```python
from build123d import *
from OCP.BRepFilletAPI import BRepFilletAPI_MakeFillet

# Parameters (mm, degrees)
ESQUISSE1_W             = 23
ESQUISSE1_H             = 20
BOSS_EXTRU_1_DEPTH      = 11.5
ESQUISSE2_W             = 11.5
ESQUISSE2_H             = 1.8
BOSS_EXTRU_2_DEPTH      = 4.5
BOSS_EXTRU_3_DEPTH      = 4
ENL_V_MAT_EXTRU_1_REACH = 27.382
ESQUISSE4_R             = 0.5
CONG_1_R1               = 1
CONG_1_R2               = 2
ESQUISSE5_R             = 2
BOSS_EXTRU_4_DEPTH      = 3.5


with BuildPart() as part:
    # Esquisse1 → Boss.-Extru.1 (new body)
    with BuildSketch(Plane.XY):
        Rectangle(ESQUISSE1_W, ESQUISSE1_H)
    extrude(amount=BOSS_EXTRU_1_DEPTH)

    # Esquisse2 → Boss.-Extru.2 (add)
    with BuildSketch(Plane(origin=(11.5, 0, 0), x_dir=(0, 0, -1), z_dir=(1, 0, 0))):
        with Locations((-5.75, 5.1)):
            Rectangle(ESQUISSE2_W, ESQUISSE2_H)
    boss_extru_2 = extrude(amount=BOSS_EXTRU_2_DEPTH)

    # Sym_trie1: Boss.-Extru.2 across plane
    add(boss_extru_2.mirror(Plane(origin=(0, 0, 0), x_dir=(0, 0, 1), z_dir=(1, 0, 0))))

    # Esquisse3 → Boss.-Extru.3 (add)
    with BuildSketch(Plane(origin=(0, 10, 0), x_dir=(1, 0, 0), z_dir=(0, 1, 0))):
        with BuildLine():
            Line((-0.290992678, -8.604781917), (-0.577609195, -8.604781917))
            ThreePointArc((-0.577609195, -8.604781917), (-3.459311015, -5.723080096), (-0.577609195, -2.841378276))
            Line((-0.577609195, -2.841378276), (-0.247327135, -2.841378276))
            ThreePointArc((-0.247327135, -2.841378276), (0.608978248, -2.648791092), (1.30037019, -2.108119366))
            ThreePointArc((1.30037019, -2.108119366), (11.499942495, -5.775715864), (1.267973174, -9.351934971))
            ThreePointArc((1.267973174, -9.351934971), (0.573387477, -8.801216851), (-0.290992678, -8.604781917))
        make_face()
    extrude(amount=BOSS_EXTRU_3_DEPTH)

    # Esquisse4 → Enl_v. mat.-Extru.1 (cut, up to next)
    with BuildSketch(Plane(origin=(0, 6, 0), x_dir=(1, 0, 0), z_dir=(0, 1, 0)), mode=Mode.PRIVATE) as enl_v_mat_extru_1_sk1:
        with Locations(Location((-13.75, -5.75, 0), (0, 0, 270))):
            Circle(ESQUISSE4_R)
    enl_v_mat_extru_1_tool1 = extrude(enl_v_mat_extru_1_sk1.sketch, amount=-ENL_V_MAT_EXTRU_1_REACH, mode=Mode.PRIVATE) & part.part
    enl_v_mat_extru_1 = enl_v_mat_extru_1_tool1.solids().sort_by_distance((-13.75, 6, 5.75))[0]
    add(enl_v_mat_extru_1, mode=Mode.SUBTRACT)

    # Sym_trie2: Enl_v. mat.-Extru.1 across plane
    add(enl_v_mat_extru_1.mirror(Plane(origin=(0, 0, 0), x_dir=(0, 0, 1), z_dir=(1, 0, 0))), mode=Mode.SUBTRACT)

    # Cong_1: one fillet with a radius per group of edges: ONE call of the kernel's fillet builder (fillet() takes one radius for all edges)
    cong_1_edges_1 = [part.edges().sort_by_distance(p)[0] for p in [
        (-11.5, 8, 11.5),
        (11.5, 8, 0),
        (11.5, 8, 11.5),
        (-11.5, -2.9, 0),
        (-11.5, -2.9, 11.5),
        (11.5, -2.9, 11.5),
        (-11.5, 8, 0),
        (11.5, -2.9, 0),
    ]]
    cong_1_edges_2 = [part.edges().sort_by_distance(p)[0] for p in [
        (16, 5.1, 11.5),
        (16, 5.1, 0),
        (-16, 5.1, 0),
        (-16, 5.1, 11.5),
    ]]
    cong_1 = BRepFilletAPI_MakeFillet(part.part.solid().wrapped)
    for e in cong_1_edges_1:
        cong_1.Add(CONG_1_R1, e.wrapped)
    for e in cong_1_edges_2:
        cong_1.Add(CONG_1_R2, e.wrapped)
    add(Compound.cast(cong_1.Shape()), mode=Mode.REPLACE)

    # Esquisse5 → Boss.-Extru.4 (add)
    with BuildSketch(Plane(origin=(0, 14, 0), x_dir=(1, 0, 0), z_dir=(0, 1, 0))):
        with Locations(Location((5.75, -5.75, 0), (0, 0, 90))):
            Circle(ESQUISSE5_R)
    extrude(amount=BOSS_EXTRU_4_DEPTH)


solid = part.part
```
Input: part model. Units: mm. Frame: model coordinates. A direction names the side the tool comes from. Round coordinates to 2 decimals unless told otherwise and drop trailing zeros. Loops run counter-clockwise (first coordinate to the right, second up) from the corner with the lowest first, then second, coordinate; pieces in that order, holes last.
1) Section query A-A on y = -1.25. Return the cut outline in (x, z), plus the area to 3 significant figures.
Ans:
outline: (-11.5, 1) arc R1 ccw to (-10.5, 0) - (10.5, 0) arc R1 ccw to (11.5, 1) - (11.5, 10.5) arc R1 ccw to (10.5, 11.5) - (-10.5, 11.5) arc R1 ccw to (-11.5, 10.5) - close
area: 264 mm2
2) Section query B-B on x = -2.5. Return the cut outline in (y, z), plus the area to 3 significant figures.
Ans:
outline: (-10, 0) - (10, 0) - (10, 3.58) - (14, 3.58) - (14, 7.87) - (10, 7.87) - (10, 11.5) - (-10, 11.5) - close
area: 247 mm2
3) Set-up query: faces 1 (the flat face through (-5, 10, 6)), 2 (the flat face through (10, 10, 1)), 3 (the flat face through (11.5, -3, 6)), 4 (the flat face through (4, 14, 4)), 5 (the cylindrical face through (-11.199, 8.028, 11.215)). Return all of +Z, -Z, +X, -X, +Y, -Y with unobstructed straight access to the full face (end or side cutting, diameter ignored); none if empty.
Ans:
face 1: -X, +Y
face 2: -Z, +X, +Y
face 3: +Z, -Z, +X, -Y
face 4: +Y
face 5: +Z, -X, +Y
4) Pull-direction query (X, two-part tool) for faces 6 (the cylindrical face through (13.254, 5.113, 5.685)), 7 (the flat face through (16, 5, 6)), 8 (the flat face through (10, 10, 10)); classes: released by +X, released by -X, zero draft, split by the parting line, or undercut.
Ans:
face 6: undercut
face 7: released by +X
face 8: zero draft
5) Pin query (flat end, axial travel): pin 1 (3 mm diameter, centred on y = 8, z = 4, fed in from -X); pin 2 (1.6 mm diameter, centred on x = -13, z = 3, fed in from +Y); pin 3 (1.7 mm diameter, centred on x = 8, z = 8.5, fed in from +Y). Return the tip coordinate at first contact, or that it passes through.
Ans:
pin 1: stops at x = -11.5
pin 2: stops at y = 6
pin 3: stops at y = 14
6) Material intervals for line 1 (X direction, y = 5.3, z = 5.75); line 2 (Z direction, x = 13.75, y = 4.95); line 3 (Y direction, x = 13, z = 7), sorted ascending.
Ans:
line 1: x = -16 to -14.25, -13.25 to 13.25, 14.25 to 16
line 2: z = 0 to 5.25, 6.25 to 11.5
line 3: y = 4.2 to 6
7) Section query C-C on z = 8.25. Return the cut outline in (x, y).
Ans:
outline: (-16, 4.2) - (-11.5, 4.2) - (-11.5, -10) - (11.5, -10) - (11.5, 4.2) - (16, 4.2) - (16, 6) - (11.5, 6) - (11.5, 10) - (10.93, 10) - (10.93, 14) - (-1.96, 14) - (-1.96, 10) - (-11.5, 10) - (-11.5, 6) - (-16, 6) - close
8) Section query D-D on y = 10.5. Return the cut outline in (x, z), plus the area to 3 significant figures.
Ans:
outline: (-0.58, 2.84) - (-0.25, 2.84) arc R2 cw to (1.3, 2.11) arc R5.75 ccw (long way) to (1.27, 9.35) arc R2 cw to (-0.29, 8.6) - (-0.58, 8.6) arc R2.88 ccw to start
area: 122 mm2
